Read the model definition and answer for the solid it produces. Units are mm, in the model's axes. A direction names the side the tool comes from. Round coordinates to 2 decimals unless told otherwise and drop trailing zeros. Put each result on its own line as item: value.
from build123d import *

# Parameters (mm, degrees)
ESQUISSE1_R        = 2.033472286
ESQUISSE1_R_2      = 1.995646952
ESQUISSE1_R_3      = 1.82934304
BOSS_EXTRU_1_DEPTH = 3


with BuildPart() as part:
    # Esquisse1 → Boss.-Extru.1 (new body)
    with BuildSketch(Plane.XY):
        Polygon((-54.518120274, -33.413932292), (-57.518120274, -33.413932292), (-57.518120274, -63.413932292), (-54.518120274, -63.413932292), (-54.518120274, -70.413932292), (-44.818120274, -70.413932292), (-44.818120274, -73.413932292), (-17.518120274, -73.413932292), (-17.518120274, -70.413932292), (2.481879726, -70.413932292), (2.481879726, -73.413932292), (32.481879726, -73.413932292), (42.181879726, -73.413932292), (42.181879726, -59.550988322), (45.181879726, -59.550988322), (45.181879726, -29.550988322), (42.181879726, -29.550988322), (42.181879726, -13.413932292), (45.181879726, -13.413932292), (45.181879726, 16.586067708), (42.181879726, 16.586067708), (42.181879726, 26.586067708), (29.835043292, 26.586067708), (5.181879726, 26.586067708), (5.181879726, 23.586067708), (-14.818120274, 23.586067708), (-14.818120274, 26.586067708), (-44.818120274, 26.586067708), (-44.818120274, 23.586067708), (-54.518120274, 23.586067708), (-54.518120274, 16.586067708), (-57.518120274, 16.586067708), (-57.518120274, -13.413932292), (-54.518120274, -13.413932292), align=None)
        with Locations((-41.652875269, -23.413932292)):
            Circle(ESQUISSE1_R, mode=Mode.SUBTRACT)
        with Locations((-35.998542238, -23.413932292)):
            Circle(ESQUISSE1_R_2, mode=Mode.SUBTRACT)
        with Locations((-30.843120944, -23.413932292)):
            Circle(ESQUISSE1_R_3, mode=Mode.SUBTRACT)
    extrude(amount=BOSS_EXTRU_1_DEPTH)


solid = part.part
Item 1: For a pull along Y with two mould halves and no side action, classify faces 5 (the flat face through (-30, 26.586, 1)), 6 (the flat face through (42.182, -22, 1)), 7 (the flat face through (-44.818, 25, 1)), 8 (the flat face through (-50, -70.414, 1)) as pulls with the +Y half, pulls with the -Y half, needs draft (parallel to the pull), parting line crosses it, or undercut.
Derived:
face 5: pulls with the +Y half
face 6: undercut
face 7: needs draft
face 8: pulls with the -Y half
Item 2: Flat-ended cylindrical pins translate along their axes: pin 1 Ø1.5 at (y, z) = (25.5, 1.5) entering from -X; pin 2 Ø1.5 at (x, z) = (43.5, 1.5) entering from +Y; pin 3 Ø1.5 at (x, z) = (-51, 1.5) entering from -Y; pin 4 Ø3.5 at (x, y) = (-41.65, -23.41) entering from +Z. Find the tip coordinate at first contact, or state that the pin passes through.
Derived:
pin 1: stops at x = -44.82
pin 2: stops at y = 16.59
pin 3: stops at y = -70.41
pin 4: passes through
Item 3: Which of the six approach directions +Z, -Z, +X, -X, +Y, -Y give full straight-line access (tool end or side, diameter ignored) to faces 1 (the flat face through (-14.818, 25, 1)), 2 (the flat face through (-56, -33.414, 1)), 3 (the flat face through (2.482, -72, 1)), 4 (the flat face through (-56, -63.414, 1))?
Derived:
face 1: +Z, -Z, +Y
face 2: +Z, -Z, -X
face 3: +Z, -Z, -Y
face 4: +Z, -Z, -X, -Y
Item 4: The part is cut by section A-A (z = 2.1). State how many separate pieces and enclosed holes the cut face has, then the cut area to 3 significant figures.
Derived:
separate pieces: 1
enclosed holes: 3
area: 9,820 mm^2
Item 5: Find the intervals of material crossed by line 1 along Y through (x, z) = (-17, 1.25); line 2 along X through (y, z) = (-66.5, 1.4); line 3 along Y through (x, z) = (-31.5, 1.35), in increasing order.
Derived:
line 1: y = -70.41 to 26.59
line 2: x = -54.52 to 42.18
line 3: y = -73.41 to -25.12, -21.71 to 26.59
